Read the model definition and answer for the solid it produces. Units are mm, in the model's axes. A direction names the side the tool comes from. Coordinates: 2 decimals unless noted, no trailing zeros. Order: outer loops, then holes, each group sorted by start corner. A loop starts at its lowest first (then second) coordinate and runs counter-clockwise, first axis right, second up. Notation, with made-up numbers: M 1,-14 L 36,-14 A4 ccw 36,-7 Z; hole C -5.75,16.5 d9. An arc over 180 degrees is marked long. Put each result on its own line as item: value.
from build123d import *

# Parameters (mm, degrees)
SKETCH1_W           = 10
SKETCH1_H           = 5
SKETCH1_W_2         = 16
SKETCH1_H_2         = 4
BOSS_EXTRUDE1_DEPTH = 194.5
SKETCH2_W           = 6.1
SKETCH2_H           = 6.1
CUT_EXTRUDE1_DEPTH  = 20


with BuildPart() as part:
    # Sketch1 → Boss-Extrude1 (new body)
    with BuildSketch(Plane(origin=(0, 0, 0), x_dir=(0, 1, 0), z_dir=(0, 0, 1))):
        with Locations((0, -4.5)):
            Rectangle(SKETCH1_W, SKETCH1_H)
        Rectangle(SKETCH1_W_2, SKETCH1_H_2)
    extrude(amount=-BOSS_EXTRUDE1_DEPTH)

    # Sketch2 → Cut-Extrude1 (cut)
    with BuildSketch(Plane(origin=(0, 0, -194.5), x_dir=(1, 0, 0), z_dir=(0, 0, -1))):
        with Locations((2.5, 0)):
            Rectangle(SKETCH2_W, SKETCH2_H)
    extrude(amount=-CUT_EXTRUDE1_DEPTH, mode=Mode.SUBTRACT)


solid = part.part
Q1. Consider line 1 along Y through (x, z) = (5, -176.5); line 2 along Y through (x, z) = (5.5, -170); line 3 along X through (y, z) = (7, -168.5). Determine where each line is inside the solid, lowest interval first.
Answers below:
line 1: y = -5 to -3.05, 3.05 to 5
line 2: y = -5 to 5
line 3: x = -2 to 2
Q2. A tool of negligible diameter and unlimited length cuts with its end or side. For faces 5 (the face through (2, 0, -174.5)), 6 (the face through (5, -5, -96)), 7 (the face through (2, 6, -96)), from which of +Z, -Z, +X, -X, +Y, -Y can it reach the whole face along a straight path? Write none if from no direction.
Answers below:
face 5: -Z
face 6: +Z, -Z, +X, -Y
face 7: +Z, -Z, +X, +Y
Q3. Given pin 1 (4 mm diameter, centred on x = 4.5, z = -140.5, fed in from -Y); pin 2 (0.9 mm diameter, centred on y = 7, z = -101, fed in from +X); pin 3 (1.5 mm diameter, centred on x = 4, y = 1.5, fed in from -Z), each flat-ended and moving along its own axis, determine where each tip first touches the part or whether it passes through.
Answers below:
pin 1: stops at y = -5
pin 2: stops at x = 2
pin 3: stops at z = -174.5
Q4. Find section A-A on x = 4. Write down the section's boundary in (y, z), plus the area to 3 significant figures.
Answers below:
outline: M -5,-194.5 L -3.05,-194.5 L -3.05,-174.5 L 3.05,-174.5 L 3.05,-194.5 L 5,-194.5 L 5,0 L -5,0 Z
area: 1,820 mm^2
Q5. Find section B-B on z = -122.5. Write down the section's boundary in (x, y).
Answers below:
outline: M -2,-8 L 2,-8 L 2,-5 L 7,-5 L 7,5 L 2,5 L 2,8 L -2,8 Z
Q6. For a pull along Y with two mould halves and no side action, classify faces 1 (the face through (-0.55, 0, -185)), 2 (the face through (5.55, 0, -185)), 3 (the face through (1, 0, 0)), 4 (the face through (0, 8, -96)) as +Y half, -Y half, draft (parallel to the pull), parting line (faces both ways), or undercut.
Answers below:
face 1: undercut
face 2: undercut
face 3: draft
face 4: +Y half
